Autodesk Inventor part; units mm, degrees
ref_plane "YZ Plane" through (0, 0, 0) normal (1, 0, 0) x (0, 1, 0)
ref_plane "XZ Plane" through (0, 0, 0) normal (0, 1, 0) x (-1, 0, 0)
ref_plane "XY Plane" through (0, 0, 0) normal (0, 0, 1) x (1, 0, 0)
sketch "スケッチ1" plane through (0, 0, 0) normal (0, 1, 0) x (-1, 0, 0)
  line L0 (22, 39.15) -> (-22, 39.15)
  line L1 (-22, 39.15) -> (-22, -39.15)
  line L2 (-22, -39.15) -> (22, -39.15)
  line L3 (22, -39.15) -> (22, 39.15)
  line L4 (22, 39.15) -> (-22, -39.15) construction
  line L5 (-22, 39.15) -> (22, -39.15) construction
  line L6 (0, -54.81) -> (0, 54.81) construction
  line L7 (30.8, 0) -> (-30.8, 0) construction
  circle A0 centre (0, 34) radius 1.65
  circle A1 centre (0, -34) radius 1.65
  circle A2 centre (0, 17.5) radius 3.075
  circle A3 centre (0, -17.5) radius 3.075
  circle A4 centre (0, 34) radius 3
  circle A5 centre (0, -34) radius 3
  line L8 (-4.5, 39.15) -> (-4.5, -39.15)
  line L9 (4.5, 39.15) -> (4.5, -39.15)
  point P0 (0, 0)
  dimension "d0" = 3.3
  dimension "d2" = 44
  dimension "d3" = 78.3
  dimension "d4" = 68
  dimension "d7" = 6.15
  dimension "d8" = 35
  dimension "d9" = 6
  dimension "d14" = 17.5
extrude "押し出し1" add sketch "スケッチ1" along normal blind 5 contours L3 L2 L9 L0 | L9 L2 L8 L0 | L8 L2 L1 L0 | A2 | A3 | A4 | A5
extrude "押し出し2" cut sketch "スケッチ1" along normal blind 3 contours A2 | A3
extrude "押し出し3" cut sketch "スケッチ1" along normal blind 3 contours A0 | A1 | A4 | A5
extrude "押し出し4" cut sketch "スケッチ1" along normal blind 1 contours L3 L2 L9 L0 | L8 L2 L1 L0
properties part number "plathomeusbhub"
For this review, take the finished solid that the model builds, in its own axes (mm). A direction names the side the tool comes from. Coordinates: 2 decimals unless noted, no trailing zeros. Loops run counter-clockwise (first coordinate to the right, second up) from the corner with the lowest first, then second, coordinate; pieces in that order, holes last. Notation, with made-up numbers: (54, 38) - (65, 38) arc R31 ccw to (65, 69) - close; hole circle Ø8 at (22, -22.75). An arc over 180 degrees is marked (long way). Use a Markdown table: item, result. Add a question column.
Item 1: For line 1 (Z direction, x = 0, y = 0.7) (3 decimals); line 2 (Z direction, x = 0, y = 4.05); line 3 (Z direction, x = 1, y = 3.8), list the stretches that pass through material, from the lowest coordinate up.
Item 2: We need section C-C (y = 2.25). Give the boundary of the cut face in (x, z) (3 decimals), and give its area (3 significant figures).
Item 3: Tool access review of faces 1 (the face through (13, 1, 1)), 2 (the face through (0, 3, 18)), 3 (the face through (-13, 1, 1)): name each direction out of +Z, -Z, +X, -X, +Y, -Y from which nothing blocks a thin tool from reaching the whole face with its end or side.
Item 4: We need section B-B (x = 0). Give the boundary of the cut face in (y, z) (3 decimals), and give its area (3 significant figures).
Item 5: We need section A-A (z = 34). Give the boundary of the cut face in (x, y).
Item 6: We need section D-D (z = -17.5). Give the boundary of the cut face in (x, y) (3 decimals), and give its area (3 significant figures).
Item 7: Insertion check: pin 1 Ø5 at (x, z) = (-14.5, 13.5) entering from -Y; pin 2 Ø1.8 at (x, z) = (-0.5, 18.5) entering from -Y; pin 3 Ø0.8 at (y, z) = (0.5, 18) entering from +X. Each pin has a flat end and moves straight along its axis. Give the tip position at first contact, or say it passes through.
Item 8: Mouldability with a two-part tool opening along X and no side actions: class faces 4 (the face through (0, 0, 1)), 5 (the face through (-1.419, 1.479, -14.772)), 6 (the face through (-22, 3, -1)) as pulls with the +X half, pulls with the -X half, needs draft (parallel to the pull), parting line crosses it, or undercut.
Results list:
| question | item | result |
|---|---|---|
| 1 | line 1 | z = -39.15 to -37, -31 to -20.575, -14.425 to 14.425, 20.575 to 31, 37 to 39.15 |
| 1 | line 2 | z = -39.15 to -35.65, -32.35 to 32.35, 35.65 to 39.15 |
| 1 | line 3 | z = -39.15 to -35.31, -32.69 to 32.69, 35.31 to 39.15 |
| 2 | outline | (-22, -39.15) - (22, -39.15) - (22, 39.15) - (-22, 39.15) - close; hole circle Ø6.15 at (0, -17.5); hole circle Ø6.15 at (0, 17.5); hole circle Ø6 at (0, -34); hole circle Ø6 at (0, 34) |
| 2 | area | 3,330 mm^2 |
| 3 | face 1 | +Z, -Z, +X, -Y |
| 3 | face 2 | -Y |
| 3 | face 3 | +Z, -Z, -X, -Y |
| 4 | outline | (0, -39.15) - (5, -39.15) - (5, -35.65) - (3, -35.65) - (3, -37) - (0, -37) - close; (0, -31) - (3, -31) - (3, -32.35) - (5, -32.35) - (5, 32.35) - (3, 32.35) - (3, 31) - (0, 31) - (0, 20.575) - (3, 20.575) - (3, 14.425) - (0, 14.425) - (0, -14.425) - (3, -14.425) - (3, -20.575) - (0, -20.575) - close; (0, 37) - (3, 37) - (3, 35.65) - (5, 35.65) - (5, 39.15) - (0, 39.15) - close |
| 4 | area | 305 mm^2 |
| 5 | outline | (-22, 1) - (-4.5, 1) - (-4.5, 0) - (-3, 0) - (-3, 3) - (-1.65, 3) - (-1.65, 5) - (-22, 5) - close; (1.65, 3) - (3, 3) - (3, 0) - (4.5, 0) - (4.5, 1) - (22, 1) - (22, 5) - (1.65, 5) - close |
| 6 | outline | (-22, 1) - (-4.5, 1) - (-4.5, 0) - (-3.075, 0) - (-3.075, 3) - (3.075, 3) - (3.075, 0) - (4.5, 0) - (4.5, 1) - (22, 1) - (22, 5) - (-22, 5) - close |
| 6 | area | 167 mm^2 |
| 7 | pin 1 | stops at y = 1 |
| 7 | pin 2 | stops at y = 3 |
| 7 | pin 3 | stops at x = 4.5 |
| 8 | face 4 | needs draft |
| 8 | face 5 | undercut |
| 8 | face 6 | pulls with the -X half |
